For this review, take the finished solid that the model builds, in its own axes (mm). A direction names the side the tool comes from. Round coordinates to 2 decimals unless told otherwise and drop trailing zeros. Order: outer loops, then holes, each group sorted by start corner. A loop starts at its lowest first (then second) coordinate and runs counter-clockwise, first axis right, second up. Notation, with made-up numbers: (77.25, 58.5) -> (133.25, 58.5) arc R20 ccw to (133.25, 71.5) -> close; hole circle Ø7 at (68.25, 13.5). An arc over 180 degrees is marked (long way). Answer in a Markdown table with one row per item.
```python
from build123d import *

# Parameters (mm, degrees)
BASES_R                     = 4.4
BASE_DEPTH                  = 4.4
TOPBORES_R                  = 1.4
TOP_BORE_DEPTH              = 8.621023553
HORN_HALF_DEPTH             = 2
HORNATTACHS_R               = 0.5
HORN_ATTACH_DEPTH           = 18.821616088
HA_LP_COUNT                 = 3
HA_LP_PITCH                 = 2.5
HORN_BODIES_COPY_1_SKETCH_R = 0.5
HORN_BODIES_COPY_1_DEPTH    = 18.821616088
HORN_BODIES_COPY_2_SKETCH_R = 0.5
HORN_BODIES_COPY_2_DEPTH    = 18.821616088
TOOTH_DEPTH                 = 3
TOOTH_CP_COUNT              = 26
BOTTOMBORES_R               = 2.6
BOTTOM_BORE_DEPTH           = 3
TOPPOCKETCYLINDERS_R        = 3.65
TOPPOCKETCYLINDERS_R_2      = 3.15
TOP_POCKET_CYLINDER_DEPTH   = 0.5


with BuildPart() as part:
    # BaseS → BASE (new body)
    with BuildSketch(Plane(origin=(0, 0, 0), x_dir=(1, 0, 0), z_dir=(0, 1, 0))):
        with Locations(Location((0, 0, 0), (0, 0, 270))):
            Circle(BASES_R)
    extrude(amount=BASE_DEPTH)

    # TopBoreS → TOP BORE (cut, through all)
    with BuildSketch(Plane(origin=(0, 4.4, 0), x_dir=(1, 0, 0), z_dir=(0, 1, 0))):
        with Locations(Location((0, 0, 0), (0, 0, 270))):
            Circle(TOPBORES_R)
    extrude(amount=-TOP_BORE_DEPTH, mode=Mode.SUBTRACT)

    # HornHalfS → HORN HALF (add)
    with BuildSketch(Plane(origin=(0, 4.4, 0), x_dir=(1, 0, 0), z_dir=(0, 1, 0))):
        with BuildLine():
            Line((-1.063592373, 15.807540032), (-3.347342764, 2.855747962))
            ThreePointArc((-3.347342764, 2.855747962), (0, 4.4), (3.347342764, 2.855747962))
            Line((3.347342764, 2.855747962), (1.063592373, 15.807540032))
            ThreePointArc((1.063592373, 15.807540032), (0, 16.7), (-1.063592373, 15.807540032))
        make_face()
    horn_half = extrude(amount=-HORN_HALF_DEPTH)

    # HornAttachS → HORN ATTACH (cut, through all)
    with BuildSketch(Plane(origin=(0, 4.4, 0), x_dir=(1, 0, 0), z_dir=(0, 1, 0))):
        with Locations(Location((0, 15.62, 0), (0, 0, 270))):
            Circle(HORNATTACHS_R)
    horn_attach = extrude(amount=-HORN_ATTACH_DEPTH, mode=Mode.SUBTRACT)

    # HA LP: HORN ATTACH ×3
    with Locations(*[(0, 0, i * HA_LP_PITCH) for i in range(1, HA_LP_COUNT)]):
        add(horn_attach, mode=Mode.SUBTRACT)

    # HORN BODIES: HORN HALF, HORN ATTACH across plane
    add(horn_half.mirror(Plane.XY))
    add(horn_attach.mirror(Plane.XY), mode=Mode.SUBTRACT)

    # HORN BODIES copy 1 sketch → HORN BODIES copy 1 (cut, through all)
    with BuildSketch(Plane(origin=(0, 4.4, -2.5), x_dir=(1, 0, 0), z_dir=(0, 1, 0))):
        with Locations((0, -15.62)):
            Circle(HORN_BODIES_COPY_1_SKETCH_R)
    extrude(amount=-HORN_BODIES_COPY_1_DEPTH, mode=Mode.SUBTRACT)

    # HORN BODIES copy 2 sketch → HORN BODIES copy 2 (cut, through all)
    with BuildSketch(Plane(origin=(0, 4.4, -5), x_dir=(1, 0, 0), z_dir=(0, 1, 0))):
        with Locations((0, -15.62)):
            Circle(HORN_BODIES_COPY_2_SKETCH_R)
    extrude(amount=-HORN_BODIES_COPY_2_DEPTH, mode=Mode.SUBTRACT)

    # ToothS → TOOTH (cut)
    with BuildSketch(Plane.XZ):
        with BuildLine():
            Line((0, -2.9), (0.262912611, -2.586672952))
            ThreePointArc((0.262912611, -2.586672952), (0, -2.6), (-0.262912611, -2.586672952))
            Line((-0.262912611, -2.586672952), (0, -2.9))
        make_face()
    tooth = extrude(amount=-TOOTH_DEPTH, mode=Mode.SUBTRACT)

    # TOOTH CP: TOOTH ×26 about axis
    tooth_cp_axis = Axis((0, 0, 0), (0, 1, 0))
    for i in range(1, TOOTH_CP_COUNT):
        add(tooth.rotate(tooth_cp_axis, i * 360 / TOOTH_CP_COUNT), mode=Mode.SUBTRACT)

    # BottomBoreS → BOTTOM BORE (cut)
    with BuildSketch(Plane(origin=(0, 0, 0), x_dir=(-1, 0, 0), z_dir=(0, -1, 0))):
        Circle(BOTTOMBORES_R)
    extrude(amount=-BOTTOM_BORE_DEPTH, mode=Mode.SUBTRACT)

    # TopPocketCylinderS → TOP POCKET CYLINDER (add)
    with BuildSketch(Plane(origin=(0, 4.4, 0), x_dir=(1, 0, 0), z_dir=(0, 1, 0))):
        with Locations(Location((0, 0, 0), (0, 0, 270))):
            Circle(TOPPOCKETCYLINDERS_R)
        with Locations(Location((0, 0, 0), (0, 0, 270))):
            Circle(TOPPOCKETCYLINDERS_R_2, mode=Mode.SUBTRACT)
    extrude(amount=TOP_POCKET_CYLINDER_DEPTH)


solid = part.part
```
Q1. Take a section at B-B, the plane z = 13.12. Write out the cut boundary in (x, y).
Answer key:
| item | result |
|---|---|
| outline | (-1.54, 2.4) -> (-0.5, 2.4) -> (-0.5, 4.4) -> (-1.54, 4.4) -> close; (0.5, 2.4) -> (1.54, 2.4) -> (1.54, 4.4) -> (0.5, 4.4) -> close |
Q2. Take a section at D-D, the plane z = -5. Write out the cut boundary in (x, y).
Answer key:
| item | result |
|---|---|
| outline | (-2.97, 2.4) -> (2.97, 2.4) -> (2.97, 4.4) -> (-2.97, 4.4) -> close |
Q3. Take a section at A-A, the plane y = 4.1. Write out the cut boundary in (x, z), then the cut area to 3 significant figures.
Answer key:
| item | result |
|---|---|
| outline | (-3.35, -2.86) -> (-1.06, -15.81) arc R1.08 ccw to (1.06, -15.81) -> (3.35, -2.86) arc R4.4 ccw to (3.35, 2.86) -> (1.06, 15.81) arc R1.08 ccw to (-1.06, 15.81) -> (-3.35, 2.86) arc R4.4 ccw to start; hole circle Ø2.8 at (0, 0); hole circle Ø1 at (0, -15.62); hole circle Ø1 at (0, -13.12); hole circle Ø1 at (0, -10.62); hole circle Ø1 at (0, 10.62); hole circle Ø1 at (0, 13.12); hole circle Ø1 at (0, 15.62) |
| area | 153 mm^2 |
Q4. To check wall thickness, follow probe 1 along Y at (x, z) = (-2, -5); probe 2 along Y at (x, z) = (-0.75, 4); probe 3 along X at (y, z) = (3.35, -10.62). State the ranges of each line that lie inside material, in increasing order.
Answer key:
| item | result |
|---|---|
| probe 1 | y = 2.4 to 4.4 |
| probe 2 | y = 0 to 4.4 |
| probe 3 | x = -1.98 to -0.5, 0.5 to 1.98 |
Q5. The part is to be moulded in two halves that separate along Z. For faces 1 (the face through (0, 3.4, -16.7)), 2 (the face through (1.322, 1.68, 4.197)), 3 (the face through (0, 4.4, 4)), 4 (the face through (0.06, 3.71, -1.4)), say which applies: +Z half, -Z half, draft (parallel to the pull), parting line (faces both ways), or undercut.
Answer key:
| item | result |
|---|---|
| face 1 | -Z half |
| face 2 | parting line |
| face 3 | draft |
| face 4 | undercut |
Q6. Clearance check with flat-ended pins moving along their axes: pin 1 Ø1 at (x, y) = (1, 1.5) entering from -Z; pin 2 Ø2 at (x, z) = (3, 8) entering from +Y; pin 3 Ø3.5 at (x, z) = (0, -7.5) entering from -Y. State where each tip first meets the part, or that it passes through.
Answer key:
| item | result |
|---|---|
| pin 1 | stops at z = -4.37 |
| pin 2 | stops at y = 4.4 |
| pin 3 | stops at y = 2.4 |
Q7. Take a section at C-C, the plane z = 7. Write out the cut boundary in (x, y), then the cut area to 3 significant figures.
Answer key:
| item | result |
|---|---|
| outline | (-2.62, 2.4) -> (2.62, 2.4) -> (2.62, 4.4) -> (-2.62, 4.4) -> close |
| area | 10.5 mm^2 |
Q8. Tool access review of faces 5 (the face through (0.02, 3.41, -16.12)), 6 (the face through (1.4, 4.4, -0.7)): name each direction out of +Z, -Z, +X, -X, +Y, -Y from which nothing blocks a thin tool from reaching the whole face with its end or side.
Answer key:
| item | result |
|---|---|
| face 5 | +Y, -Y |
| face 6 | +Y |
